Part model, mm, in its own coordinate system. A direction names the side the tool comes from. Round coordinates to 2 decimals unless told otherwise and drop trailing zeros. Write each loop counter-clockwise with the first axis right and the second up, starting at its lowest first coordinate (ties: lowest second). Pieces come first, ordered by that corner, then holes. Notation, with made-up numbers: M 52,47.25 L 95,47.25 A30 ccw 95,78.25 Z; hole C 21.5,30 d5. An arc over 180 degrees is marked long. Use one line per item in the form item = value. Start each with the question number.
Item 1: Mould opens along X. For faces 1 (the face through (-29.97, 1.32, -7.12)), 2 (the face through (-9.31, -12.25, -3.66)), 3 (the face through (6, 0, 0)) say: +X half, -X half, draft (parallel to the pull), parting line (faces both ways), or undercut.
Item 2: Cut at B-B, the plane x = 0. State how many separate pieces and enclosed holes the cut face has, then the cut area to 3 significant figures.
Item 3: Probe L1, parallel to Y at x = 5, z = -1.5; L2, parallel to Z at x = 15, y = -25; L3, parallel to Y at x = 0, z = -4.5. List the from-to ranges inside material, lowest first.
Item 4: Which spindle directions (+Z, -Z, +X, -X, +Y, -Y) get a long thin tool onto all of the face, cutting with end or side? Do faces 4 (the face through (6, 0, -7.414)), 5 (the face through (-2.746, 0.022, -0.613)). Say none if no direction does.
Item 5: Flat gauge pins, fed straight in: pin 1 Ø9 at (x, y) = (16.24, -9.38) entering from -Z; pin 2 Ø10 at (x, y) = (-1.5, -10) entering from +Z; pin 3 Ø3.5 at (x, z) = (0, 3) entering from -Y; pin 4 Ø3 at (x, z) = (21, -5.5) entering from +Y. Where does each tip first touch, or does it go through?
Item 6: Cut at A-A, the plane z = 3. Give the cut face in (x, y).
from build123d import *

# Parameters (mm, degrees)
F0_R             = 30
F0_R_2           = 4.5
F1_DEPTH         = 7.414
F2_DEPTH         = 6
F3_R             = 1.5
F4_DEPTH         = 12.5
F5_W             = 4.6
F5_H             = 3
F6_DEPTH         = 13.414
F9_R             = 7.5
F10_DEPTH        = 25
F10_COPIES_COUNT = 6


# Not quite as in the source:
# - a pattern or mirror of a feature is missing from the dataset's text; its kind, count and spacing are read off the source's solid


with BuildPart() as f1:
    # F0 (on Top) → F1 (new body)
    with BuildSketch(Plane.XY):
        Circle(F0_R)
        Circle(F0_R_2, mode=Mode.SUBTRACT)
        Circle(F0_R_2)
    extrude(amount=-F1_DEPTH)

    # F0 (on Top) → F2 (join)
    with BuildSketch(Plane.XY):
        Circle(F0_R_2)
    extrude(amount=F2_DEPTH)

    # F3 (on Front) → F4 (cut, symmetric)
    with BuildSketch(Plane.XZ):
        with Locations((0, 3)):
            Circle(F3_R)
    extrude(amount=F4_DEPTH, both=True, mode=Mode.SUBTRACT)

    # F5 (on face) → F6 (cut, through all)
    with BuildSketch(Plane.XY.offset(6)):
        Rectangle(F5_W, F5_H)
        with BuildLine():
            ThreePointArc((-2.3, 1.5), (-2.7459060435, 0), (-2.3, -1.5))
            Line((-2.3, -1.5), (-2.3, 1.5))
        make_face()
        with BuildLine():
            Line((2.3, 1.5), (2.3, -1.5))
            ThreePointArc((2.3, -1.5), (2.745183651, 0), (2.3, 1.5))
        make_face()
    extrude(amount=-F6_DEPTH, mode=Mode.SUBTRACT)

    # F7 (on Front) → F8 (revolve, cut)
    with BuildSketch(Plane.XZ):
        Polygon((30, -3.4142135624), (30, -0.5857864376), (28.5857864376, -2), align=None)
        Polygon((30, -6.8282135624), (30, -3.9997864376), (28.5857864376, -5.414), align=None)
    revolve(axis=Axis((0, 0, 0.7614716887), (0, 0, -1)), mode=Mode.SUBTRACT)

    # F9 (on face) → F10 (cut)
    with BuildSketch(Plane.XY):
        with Locations((0, 18.75)):
            Circle(F9_R)
    f10 = extrude(amount=-F10_DEPTH, mode=Mode.SUBTRACT)

    # F10_copies: F10 ×6 about axis
    f10_copies_axis = Axis((0, 0, 0), (0, 0, 1))
    for i in range(1, F10_COPIES_COUNT):
        add(f10.rotate(f10_copies_axis, i * 360 / F10_COPIES_COUNT), mode=Mode.SUBTRACT)


solid = f1.part
Model answer:
q1.face_1 = parting line
q1.face_2 = undercut
q1.face_3 = draft
q2.separate_pieces = 6
q2.enclosed_holes = 0
q2.area = 210 mm²
q3.L1 = -28.65 to -24.34, -13.16 to 13.16, 24.34 to 28.65
q3.L2 = -7.41 to -5.98, -4.85 to -2.57, -1.43 to 0
q3.L3 = -29.5 to -26.25, -11.25 to -1.5, 1.5 to 11.25, 26.25 to 29.5
q4.face_4 = -Z, +X, -X, +Y, -Y
q4.face_5 = +Z, -Z
q5.pin_1 = through
q5.pin_2 = 0
q5.pin_3 = -4.5
q5.pin_4 = 22.1
q6.outline = M -2.3,-1.5 A2.75 cw -2.3,1.5 L -1.5,1.5 L -1.5,4.24 A4.5 ccw -1.5,-4.24 L -1.5,-1.5 Z; M 1.5,-4.24 A4.5 ccw 1.5,4.24 L 1.5,1.5 L 2.3,1.5 A2.75 cw 2.3,-1.5 L 1.5,-1.5 Z
